```python
from build123d import *

# Parameters (mm, degrees)
SKETCH_1_W            = 2.8
SKETCH_1_H            = 2.8
EXTRUDE_1_DEPTH       = 30
EXTRUDE_1_2_DEPTH     = 30
EXTRUDE_1_3_DEPTH     = 30
EXTRUDE_1_4_DEPTH     = 30
EXTRUDE_1_5_DEPTH     = 30
EXTRUDE_1_6_DEPTH     = 30
EXTRUDE_1_7_DEPTH     = 30
EXTRUDE_1_8_DEPTH     = 30
EXTRUDE_1_9_DEPTH     = 30
EXTRUDE_1_10_DEPTH    = 30
EXTRUDE_1_11_DEPTH    = 30
EXTRUDE_1_12_DEPTH    = 30
EXTRUDE_1_13_DEPTH    = 30
EXTRUDE_START         = 27
EXTRUDE_2_OUTLINE_W   = 2.8
EXTRUDE_2_OUTLINE_H   = 18.8
EXTRUDE_2_OUTLINE_W_2 = 11.7
EXTRUDE_2_OUTLINE_H_2 = 2.8
EXTRUDE_2_OUTLINE_H_3 = 21.8
EXTRUDE_2_OUTLINE_H_4 = 20
EXTRUDE_2_OUTLINE_H_5 = 12
EXTRUDE_2_DEPTH       = 3
SKETCH_2_W            = 63.2
SKETCH_2_H            = 2
CUT_EXTRUDE_1_DEPTH   = 190.900710899
SKETCH_3_W            = 11.2
SKETCH_3_H            = 3
EXTRUDE_3_DEPTH       = 2.8


# Read off the part's stored shape, not the designer's step: the extrude step
with BuildPart() as part:
    # Sketch 1 → Extrude 1 (new body)
    with BuildSketch(Plane(origin=(0, 0, 0), x_dir=(1, 0, 0), z_dir=(0, 1, 0))):
        with Locations((3, -3)):
            Rectangle(SKETCH_1_W, SKETCH_1_H)
    extrude(amount=EXTRUDE_1_DEPTH)



with BuildPart() as body_2:
    # Sketch 1 → Extrude 1 2 (new body)
    with BuildSketch(Plane(origin=(0, 0, 0), x_dir=(1, 0, 0), z_dir=(0, 1, 0))):
        with Locations((17.5, -3)):
            Rectangle(SKETCH_1_W, SKETCH_1_H)
    extrude(amount=EXTRUDE_1_2_DEPTH)


with BuildPart() as body_3:
    # Sketch 1 → Extrude 1 3 (new body)
    with BuildSketch(Plane(origin=(0, 0, 0), x_dir=(1, 0, 0), z_dir=(0, 1, 0))):
        with Locations((32, -3)):
            Rectangle(SKETCH_1_W, SKETCH_1_H)
    extrude(amount=EXTRUDE_1_3_DEPTH)


with BuildPart() as body_4:
    # Sketch 1 → Extrude 1 4 (new body)
    with BuildSketch(Plane(origin=(0, 0, 0), x_dir=(1, 0, 0), z_dir=(0, 1, 0))):
        with Locations((3, -24.6)):
            Rectangle(SKETCH_1_W, SKETCH_1_H)
    extrude(amount=EXTRUDE_1_4_DEPTH)


with BuildPart() as body_5:
    # Sketch 1 → Extrude 1 5 (new body)
    with BuildSketch(Plane(origin=(0, 0, 0), x_dir=(1, 0, 0), z_dir=(0, 1, 0))):
        with Locations((3, -49.2)):
            Rectangle(SKETCH_1_W, SKETCH_1_H)
    extrude(amount=EXTRUDE_1_5_DEPTH)


with BuildPart() as body_6:
    # Sketch 1 → Extrude 1 6 (new body)
    with BuildSketch(Plane(origin=(0, 0, 0), x_dir=(1, 0, 0), z_dir=(0, 1, 0))):
        with Locations((3, -73.8)):
            Rectangle(SKETCH_1_W, SKETCH_1_H)
    extrude(amount=EXTRUDE_1_6_DEPTH)


with BuildPart() as body_7:
    # Sketch 1 → Extrude 1 7 (new body)
    with BuildSketch(Plane(origin=(0, 0, 0), x_dir=(1, 0, 0), z_dir=(0, 1, 0))):
        with Locations((3, -98.4)):
            Rectangle(SKETCH_1_W, SKETCH_1_H)
    extrude(amount=EXTRUDE_1_7_DEPTH)


with BuildPart() as body_8:
    # Sketch 1 → Extrude 1 8 (new body)
    with BuildSketch(Plane(origin=(0, 0, 0), x_dir=(1, 0, 0), z_dir=(0, 1, 0))):
        with Locations((32, -49.2)):
            Rectangle(SKETCH_1_W, SKETCH_1_H)
    extrude(amount=EXTRUDE_1_8_DEPTH)


with BuildPart() as body_9:
    # Sketch 1 → Extrude 1 9 (new body)
    with BuildSketch(Plane(origin=(0, 0, 0), x_dir=(1, 0, 0), z_dir=(0, 1, 0))):
        with Locations((32, -24.6)):
            Rectangle(SKETCH_1_W, SKETCH_1_H)
    extrude(amount=EXTRUDE_1_9_DEPTH)


with BuildPart() as body_10:
    # Sketch 1 → Extrude 1 10 (new body)
    with BuildSketch(Plane(origin=(0, 0, 0), x_dir=(1, 0, 0), z_dir=(0, 1, 0))):
        with Locations((3, -123)):
            Rectangle(SKETCH_1_W, SKETCH_1_H)
    extrude(amount=EXTRUDE_1_10_DEPTH)


with BuildPart() as body_11:
    # Sketch 1 → Extrude 1 11 (new body)
    with BuildSketch(Plane(origin=(0, 0, 0), x_dir=(1, 0, 0), z_dir=(0, 1, 0))):
        with Locations((3, -145.8)):
            Rectangle(SKETCH_1_W, SKETCH_1_H)
    extrude(amount=EXTRUDE_1_11_DEPTH)


with BuildPart() as body_12:
    # Sketch 1 → Extrude 1 12 (new body)
    with BuildSketch(Plane(origin=(0, 0, 0), x_dir=(1, 0, 0), z_dir=(0, 1, 0))):
        with Locations((3, -168.6)):
            Rectangle(SKETCH_1_W, SKETCH_1_H)
    extrude(amount=EXTRUDE_1_12_DEPTH)


with BuildPart() as body_13:
    # Sketch 1 → Extrude 1 13 (new body)
    with BuildSketch(Plane(origin=(0, 0, 0), x_dir=(1, 0, 0), z_dir=(0, 1, 0))):
        with Locations((3, -183.4)):
            Rectangle(SKETCH_1_W, SKETCH_1_H)
    extrude(amount=EXTRUDE_1_13_DEPTH)


with BuildPart() as part_1:
    add(part.part)

    add(body_2.part)  # Extrude 2 merges body 2

    add(body_3.part)  # Extrude 2 merges body 3

    add(body_4.part)  # Extrude 2 merges body 4

    add(body_5.part)  # Extrude 2 merges body 5

    add(body_6.part)  # Extrude 2 merges body 6

    add(body_7.part)  # Extrude 2 merges body 7

    add(body_8.part)  # Extrude 2 merges body 8

    add(body_9.part)  # Extrude 2 merges body 9

    add(body_10.part)  # Extrude 2 merges body 10

    add(body_11.part)  # Extrude 2 merges body 11

    add(body_12.part)  # Extrude 2 merges body 12

    add(body_13.part)  # Extrude 2 merges body 13
    # Extrude 2 outline → Extrude 2 (add)
    with BuildSketch(Plane(origin=(0, 0, 0), x_dir=(1, 0, 0), z_dir=(0, 1, 0)).offset(EXTRUDE_START)):
        with Locations((32, -13.8)):
            Rectangle(EXTRUDE_2_OUTLINE_W, EXTRUDE_2_OUTLINE_H)
        with Locations((24.75, -3)):
            Rectangle(EXTRUDE_2_OUTLINE_W_2, EXTRUDE_2_OUTLINE_H_2)
        with Locations((10.25, -3)):
            Rectangle(EXTRUDE_2_OUTLINE_W_2, EXTRUDE_2_OUTLINE_H_2)
        with Locations((32, -36.9)):
            Rectangle(EXTRUDE_2_OUTLINE_W, EXTRUDE_2_OUTLINE_H_3)
        with Locations((3, -13.8)):
            Rectangle(EXTRUDE_2_OUTLINE_W, EXTRUDE_2_OUTLINE_H)
        with Locations((3, -36.9)):
            Rectangle(EXTRUDE_2_OUTLINE_W, EXTRUDE_2_OUTLINE_H_3)
        with Locations((3, -61.5)):
            Rectangle(EXTRUDE_2_OUTLINE_W, EXTRUDE_2_OUTLINE_H_3)
        with Locations((3, -86.1)):
            Rectangle(EXTRUDE_2_OUTLINE_W, EXTRUDE_2_OUTLINE_H_3)
        with Locations((3, -110.7)):
            Rectangle(EXTRUDE_2_OUTLINE_W, EXTRUDE_2_OUTLINE_H_3)
        with Locations((3, -134.4)):
            Rectangle(EXTRUDE_2_OUTLINE_W, EXTRUDE_2_OUTLINE_H_4)
        with Locations((3, -157.2)):
            Rectangle(EXTRUDE_2_OUTLINE_W, EXTRUDE_2_OUTLINE_H_4)
        with Locations((3, -176)):
            Rectangle(EXTRUDE_2_OUTLINE_W, EXTRUDE_2_OUTLINE_H_5)
    extrude(amount=EXTRUDE_2_DEPTH)

    # Sketch 2 → Cut-Extrude 1 (cut, through all)
    with BuildSketch(Plane.ZY.offset(-1.6)):
        with Locations((153.2, 1)):
            Rectangle(SKETCH_2_W, SKETCH_2_H)
    extrude(amount=-CUT_EXTRUDE_1_DEPTH, mode=Mode.SUBTRACT)

    # Sketch 3 → Extrude 3 (add)
    with BuildSketch(Plane(origin=(33.4, 0, 0), x_dir=(0, 0, -1), z_dir=(1, 0, 0))):
        Polygon((-63.8, 4.7), (-61.8, 4.7), (-61.8, 27), (-61.8, 30), (-63.8, 30), align=None)
        with Locations((-56.2, 28.5)):
            Rectangle(SKETCH_3_W, SKETCH_3_H)
    extrude(amount=-EXTRUDE_3_DEPTH)


solid = part_1.part
```
Here's how the part is built. I have some questions about the finished solid (model axes, mm). A direction names the side the tool comes from. Coordinates: 2 decimals unless noted, no trailing zeros. Loops run counter-clockwise (first coordinate to the right, second up) from the corner with the lowest first, then second, coordinate; pieces in that order, holes last. Notation, with made-up numbers: (26.25, 42.25) -> (79.25, 42.25) arc R8 cw to (79.25, 49.25) -> close; hole circle Ø8 at (35.5, -18.75). An arc over 180 degrees is marked (long way). Return JSON: item names as keys, results as strings.
1) Will these pins go through, and if not, where does the flat tip stop? pin 1 (2 mm diameter, centred on x = 32.5, z = 35.5, fed in from -Y); pin 2 (1 mm diameter, centred on x = 17, y = 24, fed in from +Z); pin 3 (10 mm diameter, centred on y = 18, z = 117, fed in from -X); pin 4 (2 mm diameter, centred on x = 32.5, z = 63, fed in from -Y).
Results below:
{"pin 1": "y = 27", "pin 2": "z = 4.4", "pin 3": "x = 1.6", "pin 4": "y = 4.7"}
2) If we section it at B-B, the plane y = 17.5: Count the separate pieces of the cut face and the enclosed holes in it, then the cut area to 3 significant figures.
Results below:
{"separate pieces": "14", "enclosed holes": "0", "area": "108 mm²"}
3) I need wall thicknesses on line 1 (Z direction, x = 31, y = 1.5); line 2 (X direction, y = 16, z = 48.5); line 3 (Z direction, x = 6, y = 28.75). Which ranges of each line are inside material? Lowest first, please. Write a range as from..to.
Results below:
{"line 1": "1.6..4.4, 23.2..26, 47.8..50.6", "line 2": "1.6..4.4, 30.6..33.4", "line 3": "1.6..4.4"}
4) If we section it at C-C, the plane x = 21: Write out the boundary of the cut face in (y, z), then the cut area to 3 significant figures.
Results below:
{"outline": "(27, 1.6) -> (30, 1.6) -> (30, 4.4) -> (27, 4.4) -> close", "area": "8.40 mm²"}
5) For faces 1 (the face through (1.6, 28, 94)), 2 (the face through (30.6, 27.3, 38.6)), which set-ups out of +Z, -Z, +X, -X, +Y, -Y let a thin tool reach every point of the face, with its end or its side?
Results below:
{"face 1": "+Z, -Z, -X, +Y, -Y", "face 2": "+Z, +Y, -Y"}
6) If we section it at A-A, the plane z = 32.5: Write out the boundary of the cut face in (x, y), then the cut area to 3 significant figures.
Results below:
{"outline": "(1.6, 27) -> (4.4, 27) -> (4.4, 30) -> (1.6, 30) -> close; (30.6, 27) -> (33.4, 27) -> (33.4, 30) -> (30.6, 30) -> close", "area": "16.8 mm²"}
